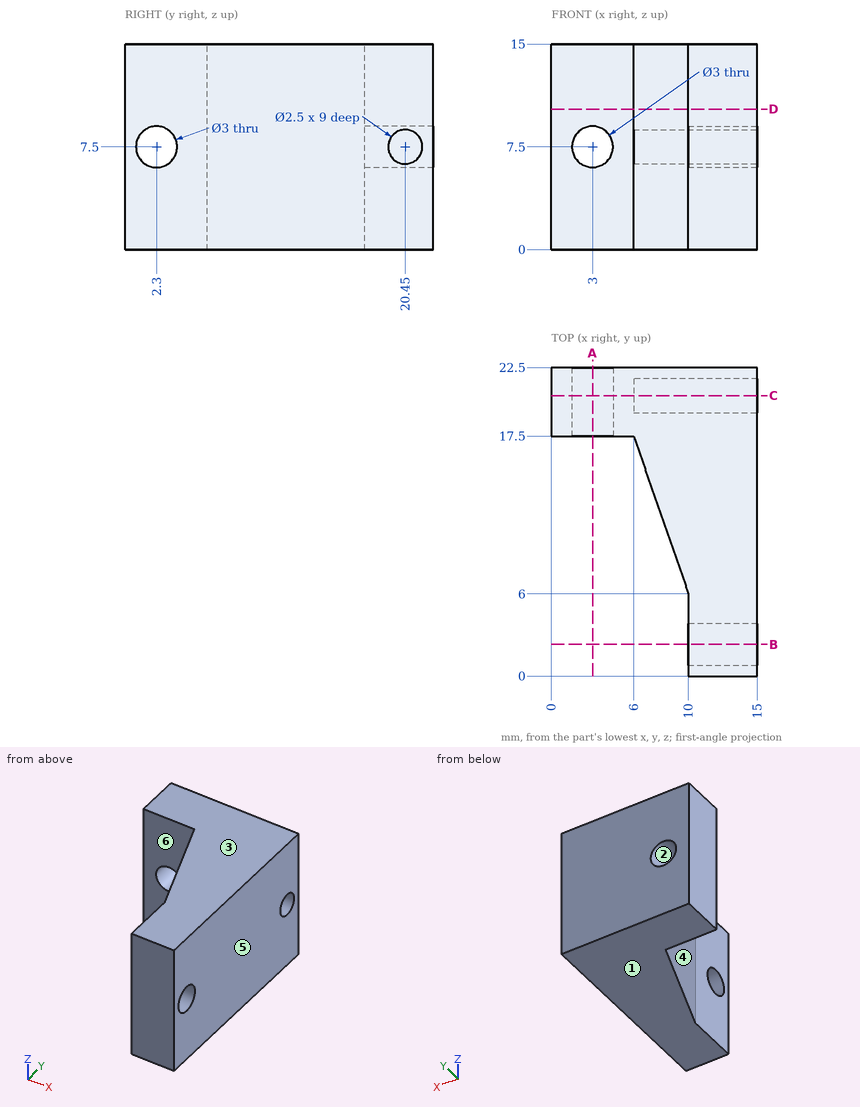
Geometry check sheet. Reference: drawing and pictorial views, mm from the part's lowest x, y, z. A direction names the side the tool comes from. Coordinates: 2 decimals unless noted, no trailing zeros. Order: outer loops, then holes, each group sorted by start corner. A loop starts at its lowest first (then second) coordinate and runs counter-clockwise, first axis right, second up.
Item 1: Section check A-A, the plane x = 3. Enter the section's corners in (y, z).
Filled in:
outline: (17.5, 0) - (22.5, 0) - (22.5, 6) - (17.5, 6) - close; (17.5, 9) - (22.5, 9) - (22.5, 15) - (17.5, 15) - close
Item 2: Material ranges on L1, parallel to Z at x = 13.85, y = 2.3; L2, parallel to X at y = 21.4, z = 7.5; L3, parallel to X at y = 1.75, z = 1.25, recorded low to high.
Filled in:
L1: z = 0 to 6, 9 to 15
L2: x = 0 to 1.5, 4.5 to 6
L3: x = 10 to 15
Item 3: Section check C-C, the plane y = 20.45. Enter the section's corners in (x, z), then the cut area to 3 significant figures.
Filled in:
outline: (0, 0) - (15, 0) - (15, 6.25) - (6, 6.25) - (6, 8.75) - (15, 8.75) - (15, 15) - (0, 15) - close; hole circle Ø3 at (3, 7.5)
area: 195 mm2
Item 4: Depth check by flat-ended pin: pin 1 (2 mm diameter, centred on y = 3.5, z = 1.5, fed in from -X); pin 2 (2.5 mm diameter, centred on x = 3, z = 7.5, fed in from +Y); pin 3 (2 mm diameter, centred on y = 20.45, z = 7.5, fed in from +X); pin 4 (3 mm diameter, centred on x = 4, z = 10.5, fed in from -Y). Enter the tip coordinate at first touch or a pass-through.
Filled in:
pin 1: stops at x = 10
pin 2: passes through
pin 3: stops at x = 6
pin 4: stops at y = 17.5
Item 5: Section check B-B, the plane y = 2.3. Enter the section's corners in (x, z).
Filled in:
outline: (10, 0) - (15, 0) - (15, 6) - (10, 6) - close; (10, 9) - (15, 9) - (15, 15) - (10, 15) - close
Item 6: Section check D-D, the plane z = 10.25. Enter the section's corners in (x, y).
Filled in:
outline: (0, 17.5) - (6, 17.5) - (10, 6) - (10, 0) - (15, 0) - (15, 22.5) - (0, 22.5) - close
Item 7: Access from +Z, -Z, +X, -X, +Y, -Y to the whole of each face (thin tool, end or side, straight path). Record for the marked faces 5 and 6.
Filled in:
face 5: +Z, -Z, +X, +Y, -Y
face 6: +Z, -Z, -X, -Y
Item 8: Release check for a two-part mould opening along Z. For the marked faces 1, 2, 3 and 4 record: +Z half, -Z half, draft (parallel to the pull), parting line (faces both ways), or undercut.
Filled in:
face 1: -Z half
face 2: undercut
face 3: +Z half
face 4: draft
